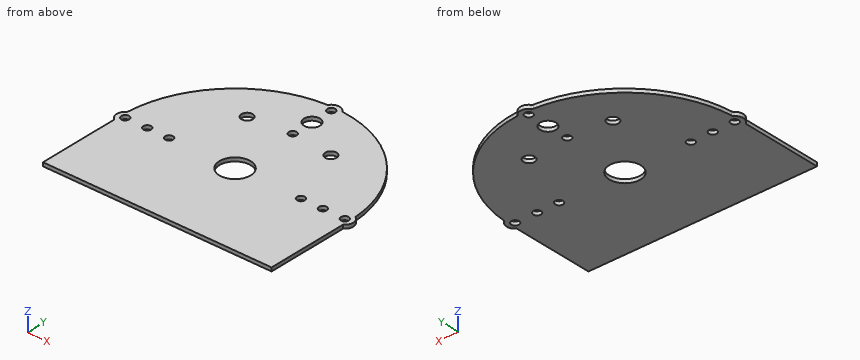
```python
from build123d import *

# Parameters (mm, degrees)
F0_R     = 8.631475
F0_R_2   = 8.6
F0_R_3   = 34.5
F0_R_4   = 12.5
F0_R_5   = 17.5
F1_DEPTH = 8


# Not quite as in the source:
# - ends of sketch curves that miss each other by under 0.0002 mm in the source are joined


with BuildPart() as f1:
    # F0 (on Top) → F1 (new body)
    with BuildSketch(Plane.XY):
        with BuildLine():
            ThreePointArc((18.476772036, 219.2230704901), (16.4501234267, 219.819241628), (14.8505619493, 221.1991429618))
            ThreePointArc((14.8505619493, 221.1991429618), (3.011e-07, 228.6), (-14.8505617308, 221.1991435511))
            ThreePointArc((-14.8505617308, 221.1991435511), (-16.4501227245, 219.8192420107), (-18.4767710413, 219.2230705631))
            ThreePointArc((-18.4767710413, 219.2230705631), (-178.5444622496, 145.9444622496), (-251.8230706896, -14.1232289494))
            ThreePointArc((-251.8230706896, -14.1232289494), (-252.4192420107, -16.1498772755), (-253.7991434425, -17.7494384132))
            ThreePointArc((-253.7991434425, -17.7494384132), (-261.1967885287, -32.2543753223), (-254.343219804, -47.0241737592))
            ThreePointArc((-254.343219804, -47.0241737592), (-252.9842553662, -48.7550030017), (-252.5, -50.90164))
            Line((-252.5, -50.90164), (-252.5, -228.6))
            Line((-252.5, -228.6), (252.5, -228.6))
            Line((252.5, -228.6), (252.5, -48.346429))
            ThreePointArc((252.5, -48.346429), (261.1975992169, -32.3011633084), (251.9889742877, -16.5436255081))
            ThreePointArc((251.9889742877, -16.5436255081), (179.4001497018, 145.0846540559), (18.476772036, 219.2230704901))
        make_face()
        with Locations((-242.6, -32.6)):
            Circle(F0_R, mode=Mode.SUBTRACT)
        with Locations((-194, -32.6)):
            Circle(F0_R_2, mode=Mode.SUBTRACT)
        with Locations((-145.5, -32.6)):
            Circle(F0_R_2, mode=Mode.SUBTRACT)
        with Locations((0, -32.6)):
            Circle(F0_R_3, mode=Mode.SUBTRACT)
        with Locations((145.5, -32.6)):
            Circle(F0_R_2, mode=Mode.SUBTRACT)
        with Locations((194, -32.6)):
            Circle(F0_R_2, mode=Mode.SUBTRACT)
        with Locations((242.6, -32.6)):
            Circle(F0_R, mode=Mode.SUBTRACT)
        with Locations((-92.5, 103.4)):
            Circle(F0_R_4, mode=Mode.SUBTRACT)
        with Locations((0, 112.9)):
            Circle(F0_R_2, mode=Mode.SUBTRACT)
        with Locations((92.5, 103.4)):
            Circle(F0_R_4, mode=Mode.SUBTRACT)
        with Locations((0, 161.4)):
            Circle(F0_R_5, mode=Mode.SUBTRACT)
        with Locations((0, 210)):
            Circle(F0_R, mode=Mode.SUBTRACT)
    extrude(amount=F1_DEPTH)


solid = f1.part
```
CAD build for the part. Positions are in the model's coordinates, mm. Round coordinates to 2 decimals unless told otherwise and drop trailing zeros. Loops run counter-clockwise (first coordinate to the right, second up) from the corner with the lowest first, then second, coordinate; pieces in that order, holes last. Notation, with made-up numbers: M 86,29 L 97,29 A22 cw 97,43 Z; hole C 87.5,-12.5 d2. An arc over 180 degrees is marked long. Return JSON: item names as keys, results as strings. Group by question number.
(1) Saw through at D-D, the plane y = 161.4. List the corners of the cut face in (x, z).
(2) Drop flat-ended pins along their axis: P1, Ø4, axis at y = -175.5, z = 4, coming from the -X side; P2, Ø4, axis at x = 189.5, z = 4.5, coming from the +Y side; P3, Ø1.5, axis at y = -48.5, z = 3, coming from the +X side. Give the stop position or say it passes through.
(3) Wall check: probe 1 along X at (y, z) = (-72, 2); probe 2 along X at (y, z) = (116.5, 3.5); probe 3 along X at (y, z) = (-21, 0.75). Give the ranges that are in metal, low to high. Write a range as [from, to].
(4) Saw through at A-A, the plane z = 5. Give the number of separate pieces and of enclosed holes in the cut face, and give its area (3 significant figures).
(5) Saw through at C-C, the plane x = -191. List the corners of the cut face in (y, z).
Answer list:
{
 "1": {"outline": "M -161.62,0 L -17.5,0 L -17.5,8 L -161.62,8 Z; M 17.5,0 L 161.62,0 L 161.62,8 L 17.5,8 Z"},
 "2": {"P1": "x = -252.5", "P2": "y = 136.52", "P3": "x = 253.39"},
 "3": {"probe 1": "[-252.5, 252.5]", "probe 2": "[-203.78, -7.81], [7.81, 203.78]", "probe 3": "[-257.14, -32.49], [32.49, 257.14]"},
 "4": {"separate pieces": "1", "enclosed holes": "12", "area": "192,000 mm2"},
 "5": {"outline": "M -228.6,0 L -40.66,0 L -40.66,8 L -228.6,8 Z; M -24.54,0 L 132.55,0 L 132.55,8 L -24.54,8 Z"}
}
